Can you work these out from the model? Positions are in its coordinate system, mm. A direction names the side the tool comes from. Round coordinates to 2 decimals unless told otherwise and drop trailing zeros. Loops run counter-clockwise (first coordinate to the right, second up) from the corner with the lowest first, then second, coordinate; pieces in that order, holes last. Notation, with made-up numbers: M -28,-19 L -19,-19 A16 cw -19,-7 Z; hole C 36.25,56.25 d11. An arc over 180 degrees is marked long. Return JSON: item names as keys, results as strings.
```python
from build123d import *

# Parameters (mm, degrees)
SKETCH1_W           = 40
SKETCH1_H           = 40
BOSS_EXTRUDE1_DEPTH = 40
CUT_EXTRUDE1_DEPTH  = 40
CUT_EXTRUDE2_DEPTH  = 40
CUT_EXTRUDE3_DEPTH  = 40
CUT_EXTRUDE4_DEPTH  = 40


with BuildPart() as part:
    # Sketch1 → Boss-Extrude1 (new body)
    with BuildSketch(Plane.XY):
        with Locations((20, 20)):
            Rectangle(SKETCH1_W, SKETCH1_H)
    extrude(amount=BOSS_EXTRUDE1_DEPTH)

    # Sketch2 → Cut-Extrude1 (cut)
    with BuildSketch(Plane.XY.offset(40)):
        Polygon((0, 0), (20, 40), (0, 40), align=None)
    extrude(amount=-CUT_EXTRUDE1_DEPTH, mode=Mode.SUBTRACT)

    # Sketch3 → Cut-Extrude2 (cut)
    with BuildSketch(Plane.XZ):
        Polygon((0, 0), (20, 20), (20, 40), (0, 40), align=None)
    extrude(amount=-CUT_EXTRUDE2_DEPTH, mode=Mode.SUBTRACT)

    # Sketch4 → Cut-Extrude3 (cut)
    with BuildSketch(Plane.ZY.offset(-20)):
        Polygon((20, 40), (40, 0), (40, 40), align=None)
    extrude(amount=-CUT_EXTRUDE3_DEPTH, mode=Mode.SUBTRACT)

    # Sketch5 → Cut-Extrude4 (cut)
    with BuildSketch(Plane(origin=(0, 0, 0), x_dir=(1, 0, 0), z_dir=(0, -0.447213595, 0.894427191))):
        Polygon((0, 0), (40, 0), (40, 44.72135955), (20, 44.72135955), align=None)
    extrude(amount=-CUT_EXTRUDE4_DEPTH, mode=Mode.SUBTRACT)


solid = part.part
```
Q1. Suppose I cut it at B-B, the plane z = 3.5. Please give me the cut outline in (x, y), plus the area to 4 significant figures.
Results:
{"outline": "M 3.5,0 L 40,0 L 40,7 L 3.5,7 Z", "area": "255.5 mm2"}
Q2. Suppose I cut it at A-A, the plane y = 11. Please give me the cut outline in (x, z).
Results:
{"outline": "M 5.5,5.5 L 40,5.5 L 40,34.5 L 20,34.5 L 20,20 Z"}
Q3. Suppose I cut it at D-D, the plane y = 20.5. Please give me the cut outline in (x, z).
Results:
{"outline": "M 10.25,10.25 L 40,10.25 L 40,29.75 L 20,29.75 L 20,20 Z"}
Q4. Suppose I cut it at C-C, the plane x = 16. Please give me the cut outline in (y, z), plus the area to 3 significant figures.
Results:
{"outline": "M 0,0 L 32,16 L 0,16 Z", "area": "256 mm2"}
Q5. I'm going to push flat-ended pins straight in: pin 1 Ø6 at (y, z) = (25, 29) entering from -X; pin 2 Ø8 at (x, y) = (14, 8.5) entering from -Z; pin 3 Ø3 at (x, y) = (27, 14.5) entering from -Z. Where does each tip first touch, or does it pass through?
Results:
{"pin 1": "stops at x = 20", "pin 2": "stops at z = 2.25", "pin 3": "stops at z = 6.5"}
Q6. If I drill on line 1 along X through (y, z) = (2, 32); line 2 along Y through (x, z) = (28, 30); line 3 along X through (y, z) = (25.5, 17.5), over which ranges is the centre line in solid material (lowest first)?
Results:
{"line 1": "x = 20 to 40", "line 2": "y = 0 to 20", "line 3": "x = 17.5 to 40"}
Q7. On a 3-axis mill with a long thin cutter (end or side, diameter ignored), from which of +Z, -Z, +X, -X, +Y, -Y can I reach the whole of each face in a straight line? I mean faces 1 (the flat face through (40, 15, 20)), 2 (the flat face through (20, 15, 28)). Say none if no direction works.
Results:
{"face 1": "+Z, -Z, +X, +Y, -Y", "face 2": "+Z, -X, +Y, -Y"}
